Model file for the job. Use its own axes, mm. A direction names the side the tool comes from. Coordinates: 2 decimals unless noted, no trailing zeros. Order: outer loops, then holes, each group sorted by start corner. A loop starts at its lowest first (then second) coordinate and runs counter-clockwise, first axis right, second up.
from build123d import *

# Parameters (mm, degrees)
STOCK_DECKMOLD_1_DEPTH = 457.2
SKETCH1_W              = 457.2
SKETCH1_H              = 76.2
BOSS_EXTRUDE1_DEPTH    = 50.8
SKETCH2_W              = 457.2
SKETCH2_H              = 76.2
BOSS_EXTRUDE2_DEPTH    = 50.8
BOSS_EXTRUDE4_DEPTH    = 25.4
BOSS_EXTRUDE5_START    = 25.4
BOSS_EXTRUDE5_DEPTH    = 25.4


# Read off the part's stored shape, not the designer's step: Stock-deckmold-1
with BuildPart() as part:
    # Stock-deckmold-1 outline → Stock-deckmold-1 (new body)
    with BuildSketch(Plane.XY):
        with BuildLine():
            Line((304.8, 25.4), (-304.8, 25.4))
            Line((-304.8, 25.4), (-304.8, -50.8))
            ThreePointArc((-304.8, -50.8), (-289.921024484, -14.878975516), (-254, 0))
            Line((-254, 0), (254, 0))
            ThreePointArc((254, 0), (289.921024484, -14.878975516), (304.8, -50.8))
            Line((304.8, -50.8), (304.8, 25.4))
        make_face()
    extrude(amount=STOCK_DECKMOLD_1_DEPTH)

    # Sketch1 → Boss-Extrude1 (add)
    with BuildSketch(Plane(origin=(304.8, 0, 0), x_dir=(0, 0, -1), z_dir=(1, 0, 0))):
        with Locations((-228.6, -12.7)):
            Rectangle(SKETCH1_W, SKETCH1_H)
    extrude(amount=BOSS_EXTRUDE1_DEPTH)

    # Sketch2 → Boss-Extrude2 (add)
    with BuildSketch(Plane.ZY.offset(304.8)):
        with Locations((228.6, -12.7)):
            Rectangle(SKETCH2_W, SKETCH2_H)
    extrude(amount=BOSS_EXTRUDE2_DEPTH)

    # Sketch3 → Boss-Extrude4 (add)
    with BuildSketch(Plane.XY.offset(457.2)):
        with BuildLine():
            Line((355.6, -50.8), (355.6, 25.4))
            Line((355.6, 25.4), (-355.6, 25.4))
            Line((-355.6, 25.4), (-355.6, -50.8))
            Line((-355.6, -50.8), (-304.8, -50.8))
            ThreePointArc((-304.8, -50.8), (-289.921024484, -14.878975516), (-254, 0))
            Line((-254, 0), (254, 0))
            ThreePointArc((254, 0), (289.921024484, -14.878975516), (304.8, -50.8))
            Line((304.8, -50.8), (355.6, -50.8))
        make_face()
    extrude(amount=BOSS_EXTRUDE4_DEPTH)

    # Sketch4 → Boss-Extrude5 (add)
    with BuildSketch(Plane(origin=(0, 0, 0), x_dir=(-1, 0, 0), z_dir=(0, 0, -1)).offset(BOSS_EXTRUDE5_START)):
        with BuildLine():
            Line((-254, 0), (254, 0))
            ThreePointArc((254, 0), (289.921024484, -14.878975516), (304.8, -50.8))
            Line((304.8, -50.8), (355.6, -50.8))
            Line((355.6, -50.8), (355.6, 25.4))
            Line((355.6, 25.4), (-355.6, 25.4))
            Line((-355.6, 25.4), (-355.6, -50.8))
            Line((-355.6, -50.8), (-304.8, -50.8))
            ThreePointArc((-304.8, -50.8), (-289.921024484, -14.878975516), (-254, 0))
        make_face()
    extrude(amount=-BOSS_EXTRUDE5_DEPTH)


solid = part.part
Q1. Cut at B-B, the plane z = 96. List the corners of the cut face in (x, y), plus the area to 3 significant figures.
Established:
outline: (-355.6, -50.8) - (-304.8, -50.8) arc R50.8 cw to (-254, 0) - (254, 0) arc R50.8 cw to (304.8, -50.8) - (355.6, -50.8) - (355.6, 25.4) - (-355.6, 25.4) - close
area: 24,300 mm2
Q2. Which spindle directions (+Z, -Z, +X, -X, +Y, -Y) get a long thin tool onto all of the face, cutting with end or side? Do faces 1 (the face through (-289.524, -14.486, 225.044)), 2 (the face through (355.6, -12, 225)). Say none if no direction does.
Established:
face 1: +Z, -Z, -Y
face 2: +Z, -Z, +X, +Y, -Y
Q3. Probe line 1 (Y direction, x = -206, z = 169); line 2 (X direction, y = -15, z = 215.5); line 3 (X direction, y = -20, z = 188.5). List the from-to ranges inside material, lowest first.
Established:
line 1: y = 0 to 25.4
line 2: x = -355.6 to -290.04, 290.04 to 355.6
line 3: x = -355.6 to -294.4, 294.4 to 355.6
Q4. Cut at D-D, the plane x = 284. List the corners of the cut face in (y, z).
Established:
outline: (-9.8, -25.4) - (25.4, -25.4) - (25.4, 482.6) - (-9.8, 482.6) - close
Q5. Cut at A-A, the plane y = -35.5. List the corners of the cut face in (x, z).
Established:
outline: (-355.6, -25.4) - (-302.44, -25.4) - (-302.44, 482.6) - (-355.6, 482.6) - close; (302.44, -25.4) - (355.6, -25.4) - (355.6, 482.6) - (302.44, 482.6) - close
Q6. Drop a flat-ended pin along its axis: P1, Ø1, axis at x = 88.5, y = -1, coming from the +Z side. Give the stop position or say it passes through.
Established:
P1: passes through
Q7. Cut at C-C, the plane x = 158. List the corners of the cut face in (y, z).
Established:
outline: (0, -25.4) - (25.4, -25.4) - (25.4, 482.6) - (0, 482.6) - close
